Autodesk Inventor part; units mm, degrees
ref_plane "YZ Plane" through (0, 0, 0) normal (1, 0, 0) x (0, 1, 0)
ref_plane "XZ Plane" through (0, 0, 0) normal (0, 1, 0) x (-1, 0, 0)
ref_plane "XY Plane" through (0, 0, 0) normal (0, 0, 1) x (1, 0, 0)
sketch "草图1" plane through (0, 0, 0) normal (1, 0, 0) x (0, 1, 0)
  circle A0 centre (0, 0) radius 2
  dimension "孔径" = 4
extrude "拉伸1" add sketch "草图1" along normal blind 20
sketch "草图2" plane through (0, 0, 0) normal (0, 1, 0) x (-1, 0, 0)
  line L0 (-20, 2) -> (-20, -2)
  line L1 (0, -2) -> (0, 2)
  line L2 (0, 2) -> (-20, 2)
  line L3 (-4, 2) -> (-4, -2)
  line L4 (0, 0) -> (-4, 0) construction
  line L5 (0, 1.25) -> (-4, 1.25)
  line L6 (0, -1.25) -> (-4, -1.25)
  dimension "d4" = 4
  dimension "距离" = 2.5
extrude "拉伸2" cut sketch "草图2" along normal through all both and the other way through all contours L6 L3 L5 L1
sketch "草图3" plane through (0, 0, 0) normal (0, 0, 1) x (1, 0, 0)
  line L0 (4, -1.5612) -> (0, -1.5612)
  line L1 (4, -1.5612) -> (4, 1.5612)
  line L2 (0, 1.5612) -> (4, 1.5612)
  line L3 (0, -1.5612) -> (0, 1.5612)
  circle A0 centre (2, 0) radius 0.5
  point P0 (0, 0)
  dimension "销孔径" = 1
extrude "拉伸3" cut sketch "草图3" along normal through all both and the other way through all contours A0
properties part number "曲柄杆" material "木材(桦木)"
For this review, take the finished solid that the model builds, in its own axes (mm). A direction names the side the tool comes from. Round coordinates to 2 decimals unless told otherwise and drop trailing zeros. Loops run counter-clockwise (first coordinate to the right, second up) from the corner with the lowest first, then second, coordinate; pieces in that order, holes last.
(1) Mouldability with a two-part tool opening along X and no side actions: class faces 1 (the cylindrical face through (1.935, -0.496, 1.62)), 2 (the flat face through (4, 0, 0)), 3 (the flat face through (2, 1, -1.25)) as released by +X, released by -X, zero draft, split by the parting line, or undercut.
Returned:
face 1: undercut
face 2: released by -X
face 3: zero draft
(2) Tool access review of faces 4 (the flat face through (2, 1, 1.25)), 5 (the flat face through (20, 0, 0)): name each direction out of +Z, -Z, +X, -X, +Y, -Y from which nothing blocks a thin tool from reaching the whole face with its end or side.
Returned:
face 4: -X, +Y, -Y
face 5: +Z, -Z, +X, +Y, -Y
(3) We need section A-A (y = 0). Give the boundary of the cut face in (x, z).
Returned:
outline: (0, -2) - (1.5, -2) - (1.5, -1.25) - (0, -1.25) - close; (0, 1.25) - (1.5, 1.25) - (1.5, 2) - (0, 2) - close; (2.5, -2) - (20, -2) - (20, 2) - (2.5, 2) - (2.5, 1.25) - (4, 1.25) - (4, -1.25) - (2.5, -1.25) - close
(4) We need section D-D (y = -1). Give the boundary of the cut face in (x, z).
Returned:
outline: (0, -1.73) - (20, -1.73) - (20, 1.73) - (0, 1.73) - (0, 1.25) - (4, 1.25) - (4, -1.25) - (0, -1.25) - close
(5) Wall thickness on line 1 along X through (y, z) = (0, 1.6); line 2 along X through (y, z) = (-0.25, -0.4); line 3 along Z through (x, y) = (5.25, -0.1): over which ranges is each line inside the solid? List them lowest first.
Returned:
line 1: x = 0 to 1.5, 2.5 to 20
line 2: x = 4 to 20
line 3: z = -2 to 2
(6) Clearance check with flat-ended pins moving along their axes: P1, Ø0.8, axis at y = -1, z = 0, coming from the -X side; P2, Ø1.6, axis at x = 2, y = 0.5, coming from the +Z side; P3, Ø2, axis at x = 7.5, z = 1.5, coming from the +Y side. State where each tip first meets the part, or that it passes through.
Returned:
P1: stops at x = 4
P2: stops at z = 2
P3: stops at y = 1.94
(7) We need section B-B (x = 2). Give the boundary of the cut face in (y, z).
Returned:
outline: (-1.56, -1.25) arc R2 ccw to (-0.5, -1.94) - (-0.5, -1.25) - close; (-1.56, 1.25) - (-0.5, 1.25) - (-0.5, 1.94) arc R2 ccw to start; (0.5, -1.94) arc R2 ccw to (1.56, -1.25) - (0.5, -1.25) - close; (0.5, 1.25) - (1.56, 1.25) arc R2 ccw to (0.5, 1.94) - close
(8) We need section C-C (z = -1.5). Give the boundary of the cut face in (x, y), plus the area to 3 significant figures.
Returned:
outline: (0, -1.32) - (20, -1.32) - (20, 1.32) - (0, 1.32) - close; hole circle Ø1 at (2, 0)
area: 52.1 mm2
